from build123d import *

# Parameters (mm, degrees)
F0_R      = 26.5
F2_R      = 25.5
F4_R      = 18
F3_R      = 21.5
F7_W      = 13
F7_H      = 32.7027017848
F8_DEPTH  = 25
F9_START  = 1
F9_DEPTH  = 24
F7_W_2    = 1.8262825906
F7_H_2    = 8.4616364911
F10_DEPTH = 25


with BuildPart() as f5:
    # F0 (on Top) → F5 section 0
    with BuildSketch(Plane.XY):
        Circle(F0_R)
    # F2 (on offset) → F5 section 1
    with BuildSketch(Plane.XY.offset(7)):
        Circle(F2_R)
    loft()

    # F4 (on Top) → F6 section 0
    with BuildSketch(Plane.XY):
        with Locations((0, 4.5)):
            Circle(F4_R)
    # F3 (on offset) → F6 section 1
    with BuildSketch(Plane.XY.offset(7)):
        with Locations((0, 4.5)):
            Circle(F3_R)
    loft(mode=Mode.SUBTRACT)

    # F7 (on Top) → F8 (cut)
    with BuildSketch(Plane.XY):
        with Locations((0, 16.3513508924)):
            Rectangle(F7_W, F7_H)
        Polygon((-6.5, -21), (-6.5, -30), (6.5, -30), (6.5, -21), (2.5, -21), (-2.5, -21), align=None)
    extrude(amount=F8_DEPTH, mode=Mode.SUBTRACT)

    # F7 (on Top) → F9 (cut)
    with BuildSketch(Plane.XY.offset(F9_START)):
        Polygon((-2.5, -11.4733194932), (-2.5, -21), (2.5, -21), (2.5, -11.4733194932), (0.9131412953, -11.4733194932), (0.9131412953, -19.9349559844), (-0.9131412953, -19.9349559844), (-0.9131412953, -11.4733194932), align=None)
    extrude(amount=F9_DEPTH, mode=Mode.SUBTRACT)

    # F7 (on Top) → F10 (cut)
    with BuildSketch(Plane.XY):
        with Locations((0, -15.7041377388)):
            Rectangle(F7_W_2, F7_H_2)
    extrude(amount=F10_DEPTH, mode=Mode.SUBTRACT)


solid = f5.part
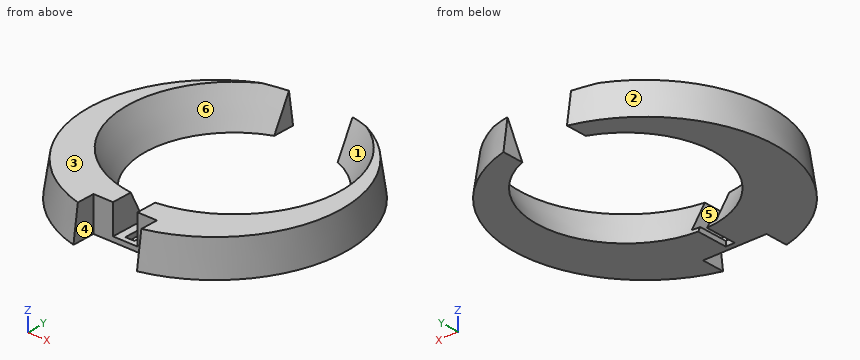
Build history of the part. All positions in model axes, mm. Face numbers are marked on the shaded views. A direction names the side the tool comes from. Coordinates: 2 decimals unless noted, no trailing zeros. Order: outer loops, then holes, each group sorted by start corner. A loop starts at its lowest first (then second) coordinate and runs counter-clockwise, first axis right, second up. Notation, with made-up numbers: (-27, -35) -> (-14, -35) arc R23 ccw to (-14, -18) -> close; hole circle Ø3 at (84.25, -7.75). An arc over 180 degrees is marked (long way). One line per item, written item: value.
(1) Probe line 1 (X direction, y = -6, z = 0.75); line 2 (X direction, y = 21, z = 3.25) (3 decimals); line 3 (Y direction, x = -18.5, z = 4.5). List the from-to ranges inside material, lowest first. Write a range as [from, to].
Checked values:
line 1: [-25.7, -15.08], [15.08, 25.7]
line 2: [-15.39, -10.625], [10.625, 15.39]
line 3: [-18.06, -3.73], [12.73, 18.06]
(2) Slice it at A-A, the plane z = 5.5. List the corners of the cut face in (x, y), plus the area to 3 significant figures.
Checked values:
outline: (-6.5, -24.88) -> (-6.5, -21) -> (-2.5, -21) -> (-2.5, -16.1) arc R20.75 cw to (-6.5, 24.21) -> (-6.5, 24.88) arc R25.71 ccw to start; (2.5, -21) -> (6.5, -21) -> (6.5, -24.88) arc R25.71 ccw to (6.5, 24.88) -> (6.5, 24.21) arc R20.75 cw to (2.5, -16.1) -> close
area: 636 mm2
(3) Tool access for the marked faces 4, 5 and 6: list every direction of +Z, -Z, +X, -X, +Y, -Y with a clear straight run to the whole face (end or side of a thin tool).
Checked values:
face 4: +Z, -Z, -Y
face 5: +Z, +Y, -Y
face 6: +Z
(4) Mould opens along Y. For the marked faces 1, 2 and 3 say: pulls with the +Y half, pulls with the -Y half, needs draft (parallel to the pull), parting line crosses it, or undercut.
Checked values:
face 1: undercut
face 2: parting line crosses it
face 3: needs draft
(5) Drop flat-ended pins along their axis: pin 1 Ø0.8 at (x, z) = (0, 0.5) entering from +Y; pin 2 Ø1.5 at (x, y) = (0.5, -17.5) entering from +Z; pin 3 Ø3 at (y, z) = (-1.5, 6) entering from -X; pin 4 Ø4 at (x, y) = (-19.5, 9) entering from -Z. Give the stop position or say it passes through.
Checked values:
pin 1: y = -19.93
pin 2: z = 1
pin 3: x = -25.83
pin 4: z = 0
(6) Slice it at B-B, the plane z = 2.5. List the corners of the cut face in (x, y), plus the area to 3 significant figures.
Checked values:
outline: (-6.5, -25.32) -> (-6.5, -21) -> (-2.5, -21) -> (-2.5, -14.59) arc R19.25 cw to (-6.5, 22.62) -> (-6.5, 25.32) arc R26.14 ccw to start; (2.5, -21) -> (6.5, -21) -> (6.5, -25.32) arc R26.14 ccw to (6.5, 25.32) -> (6.5, 22.62) arc R19.25 cw to (2.5, -14.59) -> close
area: 856 mm2
